Model file for the job. Use its own axes, mm. Face numbers are marked on the shaded views. A direction names the side the tool comes from. Round coordinates to 2 decimals unless told otherwise and drop trailing zeros. Order: outer loops, then holes, each group sorted by start corner. A loop starts at its lowest first (then second) coordinate and runs counter-clockwise, first axis right, second up. Notation, with made-up numbers: (20.5, 10) - (48.5, 10) arc R13 cw to (48.5, 24) - close; hole circle Ø11 at (7.25, 19.25). An arc over 180 degrees is marked (long way). Answer as CSV lines item,"result". Start each with the question number.
1. Band-saw the part on B-B on y = 0. List the corners of the cut face in (x, z).
2. Pin check, flat tips, straight feed: pin 1 Ø1.9 at (x, y) = (14, 1) entering from +Z; pin 2 Ø4 at (x, z) = (-2.5, -8.5) entering from +Y. Stop position of each tip, or through.
3. Pull direction Y, two halves, no side cores. Call the marked faces 1, 2 and 3: released by +Y, released by -Y, zero draft, split by the parting line, or undercut.
4. Band-saw the part on C-C on z = -1.25. List the corners of the cut face in (x, y).
5. Wall check: line 1 along Y through (x, z) = (13, -8.75); line 2 along X through (y, z) = (-0.5, -3); line 3 along X through (y, z) = (2.5, -1.25). Give the ranges that are in metal, low to high. Write a range as [from, to].
6. 3-axis set-ups, long thin cutter, end or side, ignore diameter. For the marked faces 4, 5, 6, 7 and 8: which of +Z, -Z, +X, -X, +Y, -Y reach the whole face in a straight line?
7. Band-saw the part on A-A on x = 13. List the corners of the cut face in (y, z), then the cut area to 3 significant figures.
8. Band-saw the part on D-D on z = -8.75. List the corners of the cut face in (x, y).
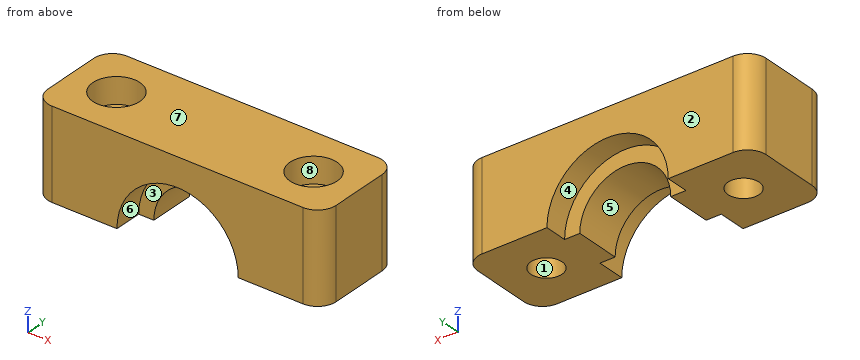
Autodesk Inventor part; units mm, degrees
ref_plane "YZ Plane" through (0, 0, 0) normal (1, 0, 0) x (0, 1, 0)
ref_plane "XZ Plane" through (0, 0, 0) normal (0, 1, 0) x (-1, 0, 0)
ref_plane "XY Plane" through (0, 0, 0) normal (0, 0, 1) x (1, 0, 0)
sketch "Base Sketch" plane through (0, 0, 0) normal (0, 0, 1) x (1, 0, 0)
  line L0 (-16.55, 6.35) -> (16.55, 6.35)
  line L1 (19, 3.9) -> (19, -3.9)
  line L2 (16.55, -6.35) -> (-16.55, -6.35)
  line L3 (-19, -3.9) -> (-19, 3.9)
  line L4 (0, 9.6004) -> (0, -9.6004) construction
  line L5 (-27.3104, 0) -> (27.3104, 0) construction
  arc A0 (19, 3.9) -> (16.55, 6.35) centre (16.55, 3.9) ccw
  arc A1 (-16.55, 6.35) -> (-19, 3.9) centre (-16.55, 3.9) ccw
  arc A2 (-19, -3.9) -> (-16.55, -6.35) centre (-16.55, -3.9) ccw
  arc A3 (16.55, -6.35) -> (19, -3.9) centre (16.55, -3.9) ccw
  point P0 (0, 0)
  point P1 (19, -6.35)
  point P2 (-19, -6.35)
  point P3 (0, 6.35)
  point P4 (19, 0)
  dimension "d0" = 38
  dimension "d2" = 2.45
  dimension "d3" = 12.7
extrude "Base Extrusion (11.75)" add sketch "Base Sketch" against normal blind 11.75
sketch "Screw Holes Sketch" plane through (0, 0, 0) normal (0, 0, 1) x (1, 0, 0)
  line L0 (0, 8.89) -> (0, -8.89) construction
  line L1 (-26.6, 0) -> (26.6, 0) construction
  circle A0 centre (-13, 0) radius 2.05
  circle A1 centre (-13, 0) radius 3.1
  circle A2 centre (13, 0) radius 2.05
  circle A3 centre (13, 0) radius 3.1
  point P0 (0, 0)
  dimension "d6" = 4.1
  dimension "d7" = 13
  dimension "d8" = 6.2
extrude "Screw Holes Extrusion (To)" cut sketch "Screw Holes Sketch" against normal up to surface (11.75 mm away) contours A0 | A2
extrude "Screw Counterbores Extrusion (3.4)" cut sketch "Screw Holes Sketch" against normal blind 3.4
sketch "Heatsink Arcs Sketch" plane through (-16.55, 6.35, 0) normal (0, 1, 0) x (1, 0, 0)
  arc A0 (10.55, 11.75) -> (22.55, 11.75) centre (16.55, 11.75) ccw
  arc A1 (8.55, 11.75) -> (24.55, 11.75) centre (16.55, 11.75) ccw
  line L0 (8.55, 11.75) -> (10.55, 11.75)
  line L1 (22.55, 11.75) -> (24.55, 11.75)
  line L2 (10.55, 11.75) -> (22.55, 11.75)
  point P0 (16.55, 0)
  dimension "d13" = 6
  dimension "d14" = 8
extrude "Top Outer Arc Extrusion (3)" cut sketch "Heatsink Arcs Sketch" against normal blind 3 contours A0 L1 A1 L0
extrude "Inner Arc Extrusion (Through)" cut sketch "Heatsink Arcs Sketch" against normal up to surface (12.7 mm away) contours L2 A0
ref_plane "Lower Outer Arc Plane (9)" through (-16.55, -2.65, 0) normal (0, 1, 0) x (1, 0, 0)
sketch "Sketch4" plane through (-16.55, -2.65, 0) normal (0, 1, 0) x (1, 0, 0)
  arc A0 (8.55, 11.75) -> (24.55, 11.75) centre (16.55, 11.75) ccw
  arc A1 (10.55, 11.75) -> (22.55, 11.75) centre (16.55, 11.75) ccw
  line L0 (22.55, 11.75) -> (24.55, 11.75)
  line L1 (8.55, 11.75) -> (10.55, 11.75)
  point P0 (16.55, 0)
extrude "Bottom Outer Arc Extrusion (3.7)" cut sketch "Sketch4" against normal up to surface (3.7 mm away)
properties part number "e3D_V6_Bowden_Clamp_01"
Reply:
1,outline,"(-19, -11.75) - (-15.05, -11.75) - (-15.05, -3.4) - (-16.1, -3.4) - (-16.1, 0) - (-19, 0) - close; (-10.95, -11.75) - (-6, -11.75) arc R6 cw to (6, -11.75) - (10.95, -11.75) - (10.95, -3.4) - (9.9, -3.4) - (9.9, 0) - (-9.9, 0) - (-9.9, -3.4) - (-10.95, -3.4) - close; (15.05, -11.75) - (19, -11.75) - (19, 0) - (16.1, 0) - (16.1, -3.4) - (15.05, -3.4) - close"
2,pin 1,"stops at z = -3.4"
2,pin 2,"stops at y = 3.35"
3,face 1,"undercut"
3,face 2,"released by +Y"
3,face 3,"released by -Y"
4,outline,"(-19, -3.9) arc R2.45 ccw to (-16.55, -6.35) - (16.55, -6.35) arc R2.45 ccw to (19, -3.9) - (19, 3.9) arc R2.45 ccw to (16.55, 6.35) - (-16.55, 6.35) arc R2.45 ccw to (-19, 3.9) - close; hole circle Ø6.2 at (-13, 0); hole circle Ø6.2 at (13, 0)"
5,line 1,"y = [-6.35, -2.05], [2.05, 6.35]"
5,line 2,"x = [-19, -16.06], [-9.94, 9.94], [16.06, 19]"
5,line 3,"x = [-19, -14.83], [-11.17, 11.17], [14.83, 19]"
6,face 4,"-Z, +Y"
6,face 5,"-Z, +Y, -Y"
6,face 6,"-Z, -Y"
6,face 7,"+Z, +X, -X, +Y, -Y"
6,face 8,"+Z"
7,outline,"(-6.35, -11.75) - (-2.05, -11.75) - (-2.05, -3.4) - (-3.1, -3.4) - (-3.1, 0) - (-6.35, 0) - close; (2.05, -11.75) - (6.35, -11.75) - (6.35, 0) - (3.1, 0) - (3.1, -3.4) - (2.05, -3.4) - close"
7,area,"93.9 mm2"
8,outline,"(-19, -3.9) arc R2.45 ccw to (-16.55, -6.35) - (-7.42, -6.35) - (-7.42, -2.65) - (-5.2, -2.65) - (-5.2, 3.35) - (-7.42, 3.35) - (-7.42, 6.35) - (-16.55, 6.35) arc R2.45 ccw to (-19, 3.9) - close; (5.2, -2.65) - (7.42, -2.65) - (7.42, -6.35) - (16.55, -6.35) arc R2.45 ccw to (19, -3.9) - (19, 3.9) arc R2.45 ccw to (16.55, 6.35) - (7.42, 6.35) - (7.42, 3.35) - (5.2, 3.35) - close; hole circle Ø4.1 at (-13, 0); hole circle Ø4.1 at (13, 0)"
